from build123d import *
from build123d.topology import SkipClean

# Parameters (mm, degrees)
SKIZZE1_R   = 11.5
SKIZZE1_R_2 = 1
BODY_DEPTH  = 14


with BuildPart() as part:
    # Skizze1 → Body (new body)
    with BuildSketch(Plane.XY):
        Circle(SKIZZE1_R)
        with Locations((-8, 0)):
            Circle(SKIZZE1_R_2, mode=Mode.SUBTRACT)
        with Locations((8, 0)):
            Circle(SKIZZE1_R_2, mode=Mode.SUBTRACT)
    extrude(amount=BODY_DEPTH)

    # Skizze2 → Rotation1 (revolve)
    with SkipClean():  # the faces are left unmerged after this step: merging them gives an invalid solid
        with BuildSketch(Plane(origin=(0, 0, 0), x_dir=(1, 0, 0), z_dir=(0, 1, 0))):
            with BuildLine():
                ThreePointArc((0, -2), (-9.5, -11.5), (0, -21))
                Line((0, -21), (0, -2))
            make_face()
            with BuildLine():
                Line((0, -2), (0, -21))
                ThreePointArc((0, -21), (6.717514421, -18.217514421), (9.5, -11.5))
                ThreePointArc((9.5, -11.5), (6.717514421, -4.782485579), (0, -2))
            make_face()
        revolve(axis=Axis((0, 0, 0), (0, 0, 1)))
    add(part.part.scale(1), mode=Mode.REPLACE)  # the faces are merged on a copy


solid = part.part
Build history of the part. All positions in model axes, mm. Give positions to 0.01 mm unless a question says otherwise; leave off trailing zeros. Write each loop counter-clockwise with the first axis right and the second up, starting at its lowest first coordinate (ties: lowest second). Pieces come first, ordered by that corner, then holes. Notation, with made-up numbers: (77, 45.25) - (123, 45.25) arc R20 ccw to (123, 73.25) - close; hole circle Ø11 at (2.25, 35). An arc over 180 degrees is marked (long way). Use one line per item in the form item = value. Start each with the question number.
1. Band-saw the part on A-A on z = 2. Write the cut outline in (x, y), plus the area to 3 significant figures.
2. Band-saw the part on B-B on x = 0. Write the cut outline in (y, z).
3. Two-plate mould, pull along X, no slides. Class faces 1 (the face through (-1.5, 11.4, 6.9)), 2 (the face through (-8, -5, 14)), 3 (the face through (9, 0, 3)), 4 (the face through (-9, 0, 3)): released by +X, released by -X, zero draft, split by the parting line, or undercut.
4. Band-saw the part on D-D on z = 12. Write the cut outline in (x, y), plus the area to 3 significant figures.
5. Probe line 1 (Z direction, x = -9, y = -4.25); line 2 (Y direction, x = -8, z = 3.5); line 3 (Y direction, x = -2.25, z = 12). List the from-to ranges inside material, lowest first. Write a range as [from, to].
6. Drop flat-ended pins along their axis: pin 1 Ø1 at (x, y) = (0.5, 5) entering from +Z; pin 2 Ø1.8 at (x, y) = (-8, 0) entering from -Z; pin 3 Ø2 at (y, z) = (-8, 5) entering from +X. Give the stop position or say it passes through.
7. Band-saw the part on C-C on y = 5.25. Write the cut outline in (x, z).
Conclusion:
q1.outline = circle Ø23 at (0, 0); hole circle Ø2 at (-8, 0); hole circle Ø2 at (8, 0)
q1.area = 409 mm²
q2.outline = (-11.5, 0) - (11.5, 0) - (11.5, 14) - (9.17, 14) arc R9.5 ccw to (-9.17, 14) - (-11.5, 14) - close
q3.face_1 = split by the parting line
q3.face_2 = zero draft
q3.face_3 = undercut
q3.face_4 = undercut
q4.outline = circle Ø23 at (0, 0)
q4.area = 415 mm²
q5.line_1 = [0, 14]
q5.line_2 = [-8.26, -1], [1, 8.26]
q5.line_3 = [-11.28, 11.28]
q6.pin_1 = 19.85
q6.pin_2 = 5.19
q6.pin_3 = 9.12
q7.outline = (-10.23, 0) - (10.23, 0) - (10.23, 14) - (7.51, 14) arc R7.92 ccw to (-7.51, 14) - (-10.23, 14) - close
